Design review of the part built by this model. Coordinates are the model's own, in mm. Give positions to 0.01 mm unless a question says otherwise; leave off trailing zeros. Write each loop counter-clockwise with the first axis right and the second up, starting at its lowest first coordinate (ties: lowest second). Pieces come first, ordered by that corner, then holes. Notation, with made-up numbers: M 84.25,73.5 L 134.25,73.5 A21 cw 134.25,108.5 Z; hole C -32.5,28 d1. An arc over 180 degrees is marked long. Use one line per item in the form item = value. Start each with the question number.
from build123d import *

# Parameters (mm, degrees)
SKETCH1_W                                    = 70
SKETCH1_H                                    = 2
BASE_FLANGE1_DEPTH                           = 70
SKETCH3_R                                    = 5
CUT_EXTRUDE1_DEPTH                           = 79.287930104
CHAMFER1_SIZE                                = 5
SKETCH4_R                                    = 1.25
CUT_EXTRUDE2_DEPTH                           = 79.287930104
CSK_FOR_M2_5_COUNTERSUNK_RAISED_HEAD_2_COUNT = 2
CSK_FOR_M2_5_COUNTERSUNK_RAISED_HEAD_2_PITCH = 8.419035512
CSK_FOR_M2_5_COUNTERSUNK_RAISED_HEAD_3_COUNT = 2
CSK_FOR_M2_5_COUNTERSUNK_RAISED_HEAD_3_PITCH = 15.556349186
CSK_FOR_M2_5_COUNTERSUNK_RAISED_HEAD_4_COUNT = 2
CSK_FOR_M2_5_COUNTERSUNK_RAISED_HEAD_4_PITCH = 20.325349715
CSK_FOR_M2_5_COUNTERSUNK_RAISED_HEAD_5_COUNT = 2
CSK_FOR_M2_5_COUNTERSUNK_RAISED_HEAD_5_PITCH = 22
CSK_FOR_M2_5_COUNTERSUNK_RAISED_HEAD_6_COUNT = 2
CSK_FOR_M2_5_COUNTERSUNK_RAISED_HEAD_6_PITCH = 20.325349715
CSK_FOR_M2_5_COUNTERSUNK_RAISED_HEAD_7_COUNT = 2
CSK_FOR_M2_5_COUNTERSUNK_RAISED_HEAD_7_PITCH = 15.556349186
CSK_FOR_M2_5_COUNTERSUNK_RAISED_HEAD_8_COUNT = 2
CSK_FOR_M2_5_COUNTERSUNK_RAISED_HEAD_8_PITCH = 8.419035512
SKETCH6_R                                    = 1.5
CUT_EXTRUDE3_DEPTH                           = 79.287930104


# Sheet-metal steps are written as plain solids
with BuildPart() as part:
    # Sketch1 → Base-Flange1 (new body)
    with BuildSketch(Plane.XY):
        with Locations((0, -1)):
            Rectangle(SKETCH1_W, SKETCH1_H)
    extrude(amount=BASE_FLANGE1_DEPTH)

    # Sketch3 → Cut-Extrude1 (cut, through all)
    with BuildSketch(Plane(origin=(0, 0, 0), x_dir=(1, 0, 0), z_dir=(0, 1, 0))):
        with Locations(Location((0, -35, 0), (0, 0, 270))):
            Circle(SKETCH3_R)
    extrude(amount=-CUT_EXTRUDE1_DEPTH, mode=Mode.SUBTRACT)

    # Chamfer1
    chamfer1_edges = [part.edges().sort_by_distance(p)[0] for p in [
        (-35, -1, 70),
        (-35, -1, 0),
        (35, -1, 0),
        (35, -1, 70),
    ]]
    chamfer(chamfer1_edges, length=CHAMFER1_SIZE)

    # Sketch4 → Cut-Extrude2 (cut, through all)
    with BuildSketch(Plane(origin=(0, 0, 0), x_dir=(1, 0, 0), z_dir=(0, 1, 0))):
        with Locations(Location((11, -35, 0), (0, 0, 270))):
            Circle(SKETCH4_R)
        with Locations(Location((-11, -35, 0), (0, 0, 270))):
            Circle(SKETCH4_R)
        with Locations(Location((0, -46, 0), (0, 0, 270))):
            Circle(SKETCH4_R)
        with Locations(Location((0, -24, 0), (0, 0, 270))):
            Circle(SKETCH4_R)
        with Locations(Location((7.778174593, -42.778174593, 0), (0, 0, 270))):
            Circle(SKETCH4_R)
        with Locations(Location((7.778174593, -27.221825407, 0), (0, 0, 270))):
            Circle(SKETCH4_R)
        with Locations(Location((-7.778174593, -27.221825407, 0), (0, 0, 270))):
            Circle(SKETCH4_R)
        with Locations(Location((-7.778174593, -42.778174593, 0), (0, 0, 270))):
            Circle(SKETCH4_R)
    extrude(amount=-CUT_EXTRUDE2_DEPTH, mode=Mode.SUBTRACT)

    # Sketch5 → CSK for M2.5 Countersunk Raised Head Screw1 (revolve, cut)
    with BuildSketch(Plane(origin=(0, -2, 46), x_dir=(0, 0, -1), z_dir=(1, 0, 0))):
        Polygon((0, 0), (0, 2), (1.45, 2), (1.45, 1.3), (2.75, 0), align=None)
    csk_for_m2_5_countersunk_raised_head_scr = revolve(axis=Axis((0, -8.35, 46), (0, 1, 0)), mode=Mode.SUBTRACT)

    # CSK for M2.5 Countersunk Raised Head 2: CSK for M2.5 Countersunk Raised Head Screw1 ×2
    with Locations(*[Vector(-0.9238795325112854, 0, -0.382683432365093) * (i * CSK_FOR_M2_5_COUNTERSUNK_RAISED_HEAD_2_PITCH) for i in range(1, CSK_FOR_M2_5_COUNTERSUNK_RAISED_HEAD_2_COUNT)]):
        add(csk_for_m2_5_countersunk_raised_head_scr, mode=Mode.SUBTRACT)

    # CSK for M2.5 Countersunk Raised Head 3: CSK for M2.5 Countersunk Raised Head Screw1 ×2
    with Locations(*[Vector(-0.7071067811865474, 0, -0.7071067811865478) * (i * CSK_FOR_M2_5_COUNTERSUNK_RAISED_HEAD_3_PITCH) for i in range(1, CSK_FOR_M2_5_COUNTERSUNK_RAISED_HEAD_3_COUNT)]):
        add(csk_for_m2_5_countersunk_raised_head_scr, mode=Mode.SUBTRACT)

    # CSK for M2.5 Countersunk Raised Head 4: CSK for M2.5 Countersunk Raised Head Screw1 ×2
    with Locations(*[Vector(-0.3826834323650891, 0, -0.9238795325112871) * (i * CSK_FOR_M2_5_COUNTERSUNK_RAISED_HEAD_4_PITCH) for i in range(1, CSK_FOR_M2_5_COUNTERSUNK_RAISED_HEAD_4_COUNT)]):
        add(csk_for_m2_5_countersunk_raised_head_scr, mode=Mode.SUBTRACT)

    # CSK for M2.5 Countersunk Raised Head 5: CSK for M2.5 Countersunk Raised Head Screw1 ×2
    with Locations(*[(0, 0, -i * CSK_FOR_M2_5_COUNTERSUNK_RAISED_HEAD_5_PITCH) for i in range(1, CSK_FOR_M2_5_COUNTERSUNK_RAISED_HEAD_5_COUNT)]):
        add(csk_for_m2_5_countersunk_raised_head_scr, mode=Mode.SUBTRACT)

    # CSK for M2.5 Countersunk Raised Head 6: CSK for M2.5 Countersunk Raised Head Screw1 ×2
    with Locations(*[Vector(0.3826834323650891, 0, -0.9238795325112871) * (i * CSK_FOR_M2_5_COUNTERSUNK_RAISED_HEAD_6_PITCH) for i in range(1, CSK_FOR_M2_5_COUNTERSUNK_RAISED_HEAD_6_COUNT)]):
        add(csk_for_m2_5_countersunk_raised_head_scr, mode=Mode.SUBTRACT)

    # CSK for M2.5 Countersunk Raised Head 7: CSK for M2.5 Countersunk Raised Head Screw1 ×2
    with Locations(*[Vector(0.7071067811865474, 0, -0.7071067811865478) * (i * CSK_FOR_M2_5_COUNTERSUNK_RAISED_HEAD_7_PITCH) for i in range(1, CSK_FOR_M2_5_COUNTERSUNK_RAISED_HEAD_7_COUNT)]):
        add(csk_for_m2_5_countersunk_raised_head_scr, mode=Mode.SUBTRACT)

    # CSK for M2.5 Countersunk Raised Head 8: CSK for M2.5 Countersunk Raised Head Screw1 ×2
    with Locations(*[Vector(0.9238795325112854, 0, -0.382683432365093) * (i * CSK_FOR_M2_5_COUNTERSUNK_RAISED_HEAD_8_PITCH) for i in range(1, CSK_FOR_M2_5_COUNTERSUNK_RAISED_HEAD_8_COUNT)]):
        add(csk_for_m2_5_countersunk_raised_head_scr, mode=Mode.SUBTRACT)

    # Sketch6 → Cut-Extrude3 (cut, through all)
    with BuildSketch(Plane(origin=(0, 0, 0), x_dir=(1, 0, 0), z_dir=(0, 1, 0))):
        with Locations(Location((-28, -7, 0), (0, 0, 270))):
            Circle(SKETCH6_R)
        with Locations(Location((0, -7, 0), (0, 0, 270))):
            Circle(SKETCH6_R)
        with Locations(Location((28, -7, 0), (0, 0, 270))):
            Circle(SKETCH6_R)
        with Locations(Location((28, -35, 0), (0, 0, 270))):
            Circle(SKETCH6_R)
        with Locations(Location((28, -63, 0), (0, 0, 270))):
            Circle(SKETCH6_R)
        with Locations(Location((0, -63, 0), (0, 0, 270))):
            Circle(SKETCH6_R)
        with Locations(Location((-28, -63, 0), (0, 0, 270))):
            Circle(SKETCH6_R)
        with Locations(Location((-28, -35, 0), (0, 0, 270))):
            Circle(SKETCH6_R)
    extrude(amount=-CUT_EXTRUDE3_DEPTH, mode=Mode.SUBTRACT)


solid = part.part
1. To check wall thickness, follow L1, parallel to X at y = -0.9, z = 7; L2, parallel to Z at x = 7, y = -0.2; L3, parallel to X at y = -0.6, z = 62. State the ranges of each line that lie inside material, in increasing order.
2. We need section C-C (z = 63). State the section outline as (x, y) points.
3. We need section B-B (x = 28). State the section outline as (y, z) points.
4. Draft analysis for pull direction X (two halves, no side actions). For faces 1 (the cylindrical face through (0.07, -0.99, 5.5)), 2 (the flat face through (0, -2, 42)), 3 (the flat face through (33, -1, 3)), state which applies: pulls with the +X half, pulls with the -X half, needs draft (parallel to the pull), parting line crosses it, or undercut.
5. We need section D-D (y = -1.5). Give the number of separate pieces and of enclosed holes in the cut face, and give its area (3 significant figures).
6. We need section A-A (z = 35). State the section outline as (x, y) points.
7. Clearance check with a flat-ended pin moving along its axis: pin 1 Ø3.5 at (x, z) = (-7.78, 42.78) entering from -Y. State where the tip first meets the part, or that it passes through.
Answer block:
q1.L1 = -35 to -29.5, -26.5 to -1.5, 1.5 to 26.5, 29.5 to 35
q1.L2 = 0 to 26, 28.45 to 41.55, 44 to 70
q1.L3 = -35 to -29.12, -26.88 to -1.12, 1.12 to 26.88, 29.12 to 35
q2.outline = M -35,-2 L -29.5,-2 L -29.5,0 L -35,0 Z; M -26.5,-2 L -1.5,-2 L -1.5,0 L -26.5,0 Z; M 1.5,-2 L 26.5,-2 L 26.5,0 L 1.5,0 Z; M 29.5,-2 L 35,-2 L 35,0 L 29.5,0 Z
q3.outline = M -2,0 L 0,0 L 0,5.5 L -2,5.5 Z; M -2,8.5 L 0,8.5 L 0,33.5 L -2,33.5 Z; M -2,36.5 L 0,36.5 L 0,61.5 L -2,61.5 Z; M -2,64.5 L 0,64.5 L 0,70 L -2,70 Z
q4.face_1 = undercut
q4.face_2 = needs draft
q4.face_3 = pulls with the +X half
q5.separate_pieces = 1
q5.enclosed_holes = 17
q5.area = 4,590 mm^2
q6.outline = M -35,-2 L -29.5,-2 L -29.5,0 L -35,0 Z; M -26.5,-2 L -13.75,-2 L -12.45,-0.7 L -12.45,0 L -26.5,0 Z; M -9.55,-0.7 L -8.25,-2 L -5,-2 L -5,0 L -9.55,0 Z; M 5,-2 L 8.25,-2 L 9.55,-0.7 L 9.55,0 L 5,0 Z; M 12.45,-0.7 L 13.75,-2 L 26.5,-2 L 26.5,0 L 12.45,0 Z; M 29.5,-2 L 35,-2 L 35,0 L 29.5,0 Z
q7.pin_1 = -1
